Input: dimensioned drawing with shaded views. Units: mm. Origin: part minimum x, y, z. A direction names the side the tool comes from. Round coordinates to 2 decimals unless told otherwise and drop trailing zeros. Loops run counter-clockwise (first coordinate to the right, second up) from the corner with the lowest first, then second, coordinate; pieces in that order, holes last. Notation, with made-up numbers: M -26.5,-1.75 L -6.5,-1.75 A22 ccw -6.5,16.25 Z; hole C -23,84 d8. An arc over 180 degrees is marked long. Use one line per item in the form item = value. Start each with the question number.
Q1. Mould query, pull axis Y, two halves, no side actions, for the marked faces 4, 5, 6 and 7. Classes: pulls with the +Y half, pulls with the -Y half, needs draft (parallel to the pull), parting line crosses it, or undercut.
Q2. Ray query, line 1 along X through (y, z) = (23.5, 14); line 2 along Y through (x, z) = (35, 37.75); line 3 along X through (y, z) = (11.5, 13). Return the intervals inside material, ascending.
Q3. Access query for the marked faces 1, 2 and 3. Directions: +Z, -Z, +X, -X, +Y, -Y. A direction counts if a zero-diameter tool reaches every point of the face in a straight line with its end or side. Return the directions, or none.
Q4. Section query A-A, the plane x = 20. Output: boundary loops of the cut face in (y, z), and give its area (3 significant figures).
Q5. Section query B-B, the plane z = 37. Output: boundary loops of the cut face in (x, y), and give its area (3 significant figures).
Q6. Section query C-C, the plane y = 20. Output: boundary loops of the cut face in (x, z), and give its area (3 significant figures).
Q7. First-contact query: P1, Ø2, axis at x = 13.5, y = 16, coming from the +Z side; P2, Ø8.5, axis at y = 20, z = 20, coming from the +X side; P3, Ø0.8, axis at x = 34.5, y = 4.5, coming from the +Z side. Flat tips, straight axial feed; report the tip coordinate or a pass-through.
Q8. Section query D-D, the plane z = 20. Output: boundary loops of the cut face in (x, y), and give its area (3 significant figures).
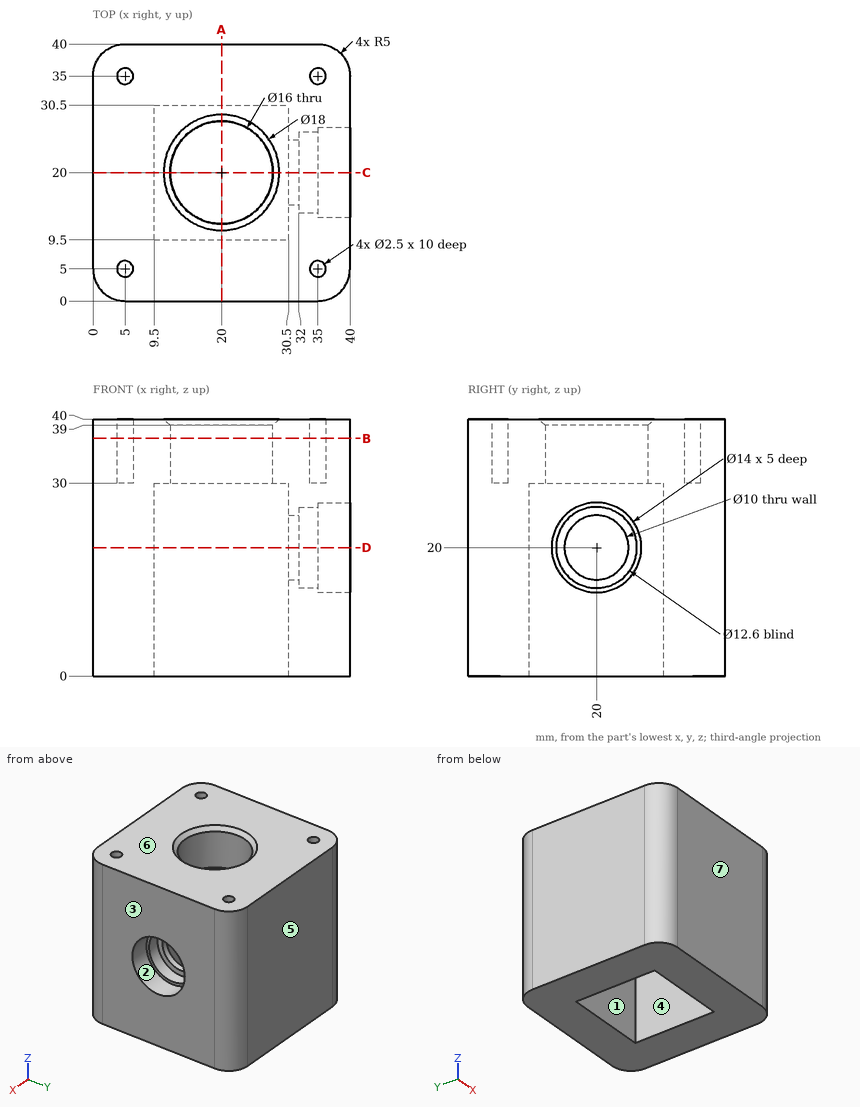
Results found:
q1.face_4 = undercut
q1.face_5 = pulls with the +Y half
q1.face_6 = needs draft
q1.face_7 = pulls with the -Y half
q2.line_1 = 0 to 9.5, 30.5 to 35
q2.line_2 = 0 to 3.75, 6.25 to 33.75, 36.25 to 40
q2.line_3 = 0 to 9.5, 30.5 to 40
q3.face_1 = -Z
q3.face_2 = +X
q3.face_3 = +Z, -Z, +X, +Y, -Y
q4.outline = M 0,0 L 9.5,0 L 9.5,30 L 12,30 L 12,39 L 11,40 L 0,40 Z; M 28,30 L 30.5,30 L 30.5,0 L 40,0 L 40,40 L 29,40 L 28,39 Z
q4.area = 809 mm²
q5.outline = M 0,5 A5 ccw 5,0 L 35,0 A5 ccw 40,5 L 40,35 A5 ccw 35,40 L 5,40 A5 ccw 0,35 Z; hole C 5,5 d2.5; hole C 5,35 d2.5; hole C 20,20 d16; hole C 35,5 d2.5; hole C 35,35 d2.5
q5.area = 1,360 mm²
q6.outline = M 0,0 L 9.5,0 L 9.5,30 L 12,30 L 12,39 L 11,40 L 0,40 Z; M 28,30 L 30.5,30 L 30.5,25 L 32,25 L 32,26.3 L 35,26.3 L 35,27 L 40,27 L 40,40 L 29,40 L 28,39 Z; M 30.5,0 L 40,0 L 40,13 L 35,13 L 35,13.7 L 32,13.7 L 32,15 L 30.5,15 Z
q6.area = 686 mm²
q7.P1 = 39.63
q7.P2 = 9.5
q7.P3 = 30
q8.outline = M 0,5 A5 ccw 5,0 L 35,0 A5 ccw 40,5 L 40,13 L 35,13 L 35,13.7 L 32,13.7 L 32,15 L 30.5,15 L 30.5,9.5 L 9.5,9.5 L 9.5,30.5 L 30.5,30.5 L 30.5,25 L 32,25 L 32,26.3 L 35,26.3 L 35,27 L 40,27 L 40,35 A5 ccw 35,40 L 5,40 A5 ccw 0,35 Z
q8.area = 1,010 mm²
